Autodesk Inventor part; units mm, degrees
ref_plane "YZ Plane" through (0, 0, 0) normal (1, 0, 0) x (0, 1, 0)
ref_plane "XZ Plane" through (0, 0, 0) normal (0, 1, 0) x (-1, 0, 0)
ref_plane "XY Plane" through (0, 0, 0) normal (0, 0, 1) x (1, 0, 0)
sketch "Sketch1" plane through (0, 0, 0) normal (0, 1, 0) x (-1, 0, 0)
  circle A0 centre (0, 0) radius 1.1684
  dimension "d0" = 2.3368
extrude "Extrusion1" add sketch "Sketch1" along normal blind 7.9375
sketch "Sketch2" plane through (0, 7.9375, 0) normal (0, 1, 0) x (1, 0, 0)
  circle A0 centre (0, 0) radius 1.1684
  circle A1 centre (0, 0) radius 2.1209
  dimension "d3" = 4.2418
extrude "Extrusion2" add sketch "Sketch2" along normal blind 1.5748 contours A0 | A1
fillet "Fillet1" radius 1.016 1 edges at (-2.1209, 9.5123, 0)
thread "Thread1"
chamfer "Chamfer1" distance 0.254 angle 45 1 edges at (1.1684, 0, 0)
sketch "Sketch3" plane through (0, 9.5123, 0) normal (0, 1, 0) x (1, 0, 0)
  circle A0 centre (0, 0) radius 1.1049
  line L0 (-0.254, -1.0753) -> (0.254, -1.0753)
  line L1 (0.254, -1.0753) -> (0.254, 1.0753)
  line L2 (0.254, 1.0753) -> (-0.254, 1.0753)
  line L3 (-0.254, 1.0753) -> (-0.254, -1.0753)
  line L4 (-1.0753, -0.254) -> (1.0753, -0.254)
  line L5 (1.0753, -0.254) -> (1.0753, 0.254)
  line L6 (1.0753, 0.254) -> (-1.0753, 0.254)
  line L7 (-1.0753, 0.254) -> (-1.0753, -0.254)
  point P0 (0, 1.0753)
  point P1 (1.0753, 0)
  dimension "d12" = 0.508
extrude "Extrusion3" cut sketch "Sketch3" against normal blind 1.27 contours L5 L4 L1 L6 | L1 L6 L3 L2 | L1 L4 L3 L6 | L0 L3 L4 L1 | L3 L4 L7 L6
properties part number "Screw"
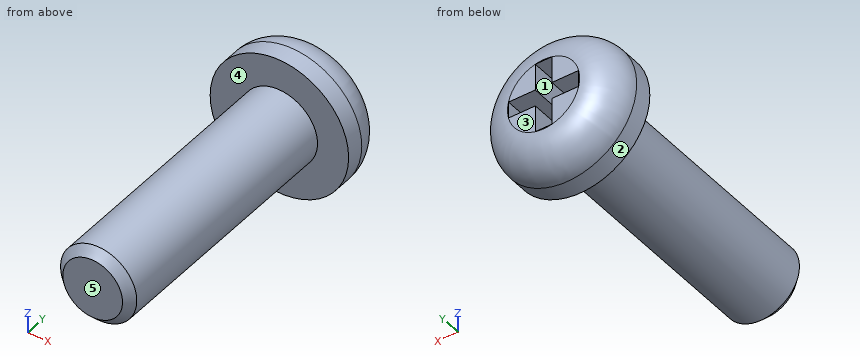
The listing builds one solid part. Answer for the finished solid, in the listing's coordinates (mm). Face numbers are marked on the shaded views. A direction names the side the tool comes from. Round coordinates to 2 decimals unless told otherwise and drop trailing zeros. Write each loop counter-clockwise with the first axis right and the second up, starting at its lowest first coordinate (ties: lowest second). Pieces come first, ordered by that corner, then holes. Notation, with made-up numbers: M 44,25.25 L 70,25.25 A24 ccw 70,36.25 Z; hole C 77,85.25 d8. An arc over 180 degrees is marked long. Write each question's results on one line, items separated by ' | '. Start each with the question number.
(1) The part is cut by section D-D, the plane y = 7.25. Write down the section's boundary in (x, z), and give its area (3 significant figures).
(2) For the marked faces 4 and 5, determine the directions among +Z, -Z, +X, -X, +Y, -Y from which every point of the face is accessible in a straight line to the end or side of a thin tool.
(3) Find the intervals of material crossed by line 1 (Z direction, x = 0, y = 4.5); line 2 (Z direction, x = -0.95, y = 9); line 3 (Y direction, x = 0.85, z = -1.1), in increasing order.
(4) The part is cut by section B-B, the plane y = 8.75. Write down the section's boundary in (x, z), and give its area (3 significant figures).
(5) Determine the mould class of the marked faces 1, 2 and 3 for opening direction Z: +Z half, -Z half, draft (parallel to the pull), parting line (faces both ways), or undercut.
(6) Each of these flat-tipped pins is pushed along its axis until it touches: P1, Ø0.7, axis at y = 9, z = -1, coming from the -X side; P2, Ø0.9, axis at y = 9, z = -0.5, coming from the +X side; P3, Ø1.5, axis at x = -0.5, y = 6.5, coming from the -Z side. Where does it stop, or does it pass through?
Worked answers:
1) outline: C 0,0 d2.34 | area: 4.29 mm²
2) face 4: -Y | face 5: +Z, -Z, +X, -X, -Y
3) line 1: z = -1.17 to 1.17 | line 2: z = -1.75 to -0.25, 0.25 to 1.75 | line 3: y = 7.94 to 9.47
4) outline: C 0,0 d4.18; hole M -1.08,-0.25 L -0.25,-0.25 L -0.25,-1.08 L 0.25,-1.08 L 0.25,-0.25 L 1.08,-0.25 L 1.08,0.25 L 0.25,0.25 L 0.25,1.08 L -0.25,1.08 L -0.25,0.25 L -1.08,0.25 Z | area: 11.8 mm²
5) face 1: undercut | face 2: parting line | face 3: draft
6) P1: stops at x = -1.95 | P2: stops at x = 2.1 | P3: stops at z = -1.17
